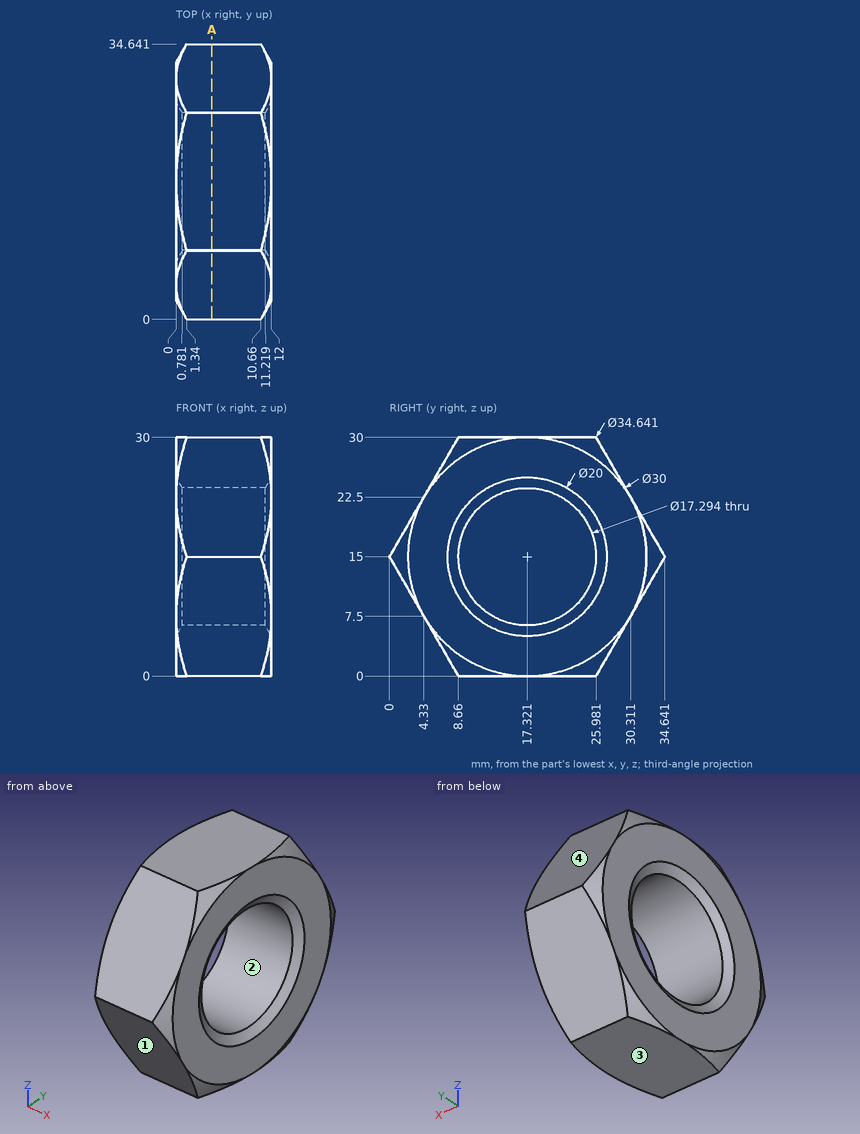
Here's the drawing with two shaded views (mm, measured from the low corner). I have some questions. Round coordinates to 2 decimals unless told otherwise and drop trailing zeros. Loops run counter-clockwise (first coordinate to the right, second up) from the corner with the lowest first, then second, coordinate; pieces in that order, holes last. Notation, with made-up numbers: (-24.75, -38) - (-19.75, -38) arc R16 cw to (-19.75, -25) - close; hole circle Ø3 at (-30.75, 18.5). An arc over 180 degrees is marked (long way). Use CSV: the item, a comma, the result in double quotes.
Item 1: I need wall thicknesses on L1, parallel to Y at x = 8.25, z = 15 (1 decimal); L2, parallel to Z at x = 8, y = 17; L3, parallel to Z at x = 3.5, y = 20. Which ranges of each line are inside material? Lowest first, please. Write a range as [from, to].
Here are the results:
L1,"y = [0, 8.7], [26, 34.6]"
L2,"z = [0, 6.36], [23.64, 30]"
L3,"z = [0, 6.78], [23.22, 30]"
Item 2: Will these pins go through, and if not, where does the flat tip stop? pin 1 (1 mm diameter, centred on x = 3, y = 29, fed in from -Z) (1 decimal); pin 2 (8 mm diameter, centred on y = 21.5, z = 22, fed in from -X); pin 3 (1 mm diameter, centred on x = 6, z = 20, fed in from -Y); pin 4 (1 mm diameter, centred on x = 7, z = 18.5, fed in from -Y).
Here are the results:
pin 1,"stops at z = 4.4"
pin 2,"stops at x = 0"
pin 3,"stops at y = 2.6"
pin 4,"stops at y = 1.73"
Item 3: If we mould it in two halves opening along Y, with no side actions, what happens to the marked faces 1, 2, 3 and 4? For each: pulls with the +Y half, pulls with the -Y half, needs draft (parallel to the pull), parting line crosses it, or undercut.
Here are the results:
face 1,"pulls with the -Y half"
face 2,"undercut"
face 3,"needs draft"
face 4,"pulls with the +Y half"
Item 4: If we section it at A-A on x = 4.5: List the corners of the cut face in (y, z) for me (1 decimal).
Here are the results:
outline,"(0, 15) - (8.7, 0) - (26, 0) - (34.6, 15) - (26, 30) - (8.7, 30) - close; hole circle Ø17.3 at (17.3, 15)"
